from build123d import *

# Parameters (mm, degrees)
SKETCH3_R                = 48
SKETCH3_R_2              = 45
BOSS_EXTRUDE1_DEPTH      = 100
BOSS_EXTRUDE2_REACH      = 150.014
BOSS_EXTRUDE2_END_RADIUS = 48
SKETCH5_R                = 10
SKETCH6_R                = 10
BOSS_EXTRUDE3_DEPTH      = 40
SKETCH7_R                = 7
CUT_EXTRUDE1_DEPTH       = 55
SKETCH8_W                = 105
SKETCH8_H                = 105
SKETCH8_R                = 45
BOSS_EXTRUDE4_DEPTH      = 3
SKETCH9_W                = 105
SKETCH9_H                = 105
SKETCH9_W_2              = 100
SKETCH9_H_2              = 100
BOSS_EXTRUDE5_DEPTH      = 10


with BuildPart() as part:
    # Sketch3 → Boss-Extrude1 (new body)
    with BuildSketch(Plane(origin=(0, 0, 0), x_dir=(1, 0, 0), z_dir=(0, 1, 0))):
        with Locations(Location((0, 0, 0), (0, 0, 270))):
            Circle(SKETCH3_R)
        with Locations(Location((0, 0, 0), (0, 0, 270))):
            Circle(SKETCH3_R_2, mode=Mode.SUBTRACT)
    extrude(amount=BOSS_EXTRUDE1_DEPTH)

    # Boss-Extrude2: up to this cylinder (the profile starts outside it)
    boss_extrude2_end = Plane(origin=(0, 26.126098, 0), z_dir=(0, -1, 0)) * Cylinder(BOSS_EXTRUDE2_END_RADIUS, 397.028, mode=Mode.PRIVATE)
    # Sketch5 → Boss-Extrude2 (add, up to the surface)
    with BuildSketch(Plane(origin=(50, 0, 0), x_dir=(0, 0, -1), z_dir=(1, 0, 0)), mode=Mode.PRIVATE) as boss_extrude2_sk1:
        with Locations((0, 26.126097613)):
            Circle(SKETCH5_R)
    boss_extrude2_tool1 = extrude(boss_extrude2_sk1.sketch, amount=-BOSS_EXTRUDE2_REACH, mode=Mode.PRIVATE) - boss_extrude2_end
    add(boss_extrude2_tool1.solids().sort_by_distance((50, 26.126098, 0))[0])

    # Sketch6 → Boss-Extrude3 (add)
    with BuildSketch(Plane(origin=(50, 0, 0), x_dir=(0, 0, -1), z_dir=(1, 0, 0))):
        with Locations(Location((0, 25.974996965, 0), (0, 0, 179.567124411))):
            Circle(SKETCH6_R)
    extrude(amount=BOSS_EXTRUDE3_DEPTH)

    # Sketch7 → Cut-Extrude1 (cut)
    with BuildSketch(Plane(origin=(90, 0, 0), x_dir=(0, 0, -1), z_dir=(1, 0, 0))):
        with Locations((0, 26.126097613)):
            Circle(SKETCH7_R)
    extrude(amount=-CUT_EXTRUDE1_DEPTH, mode=Mode.SUBTRACT)

    # Sketch8 → Boss-Extrude4 (add)
    with BuildSketch(Plane(origin=(0, 100, 0), x_dir=(1, 0, 0), z_dir=(0, 1, 0))):
        Rectangle(SKETCH8_W, SKETCH8_H)
        with Locations(Location((0, 0, 0), (0, 0, 270))):
            Circle(SKETCH8_R, mode=Mode.SUBTRACT)
    extrude(amount=BOSS_EXTRUDE4_DEPTH)

    # Sketch9 → Boss-Extrude5 (add)
    with BuildSketch(Plane(origin=(0, 103, 0), x_dir=(1, 0, 0), z_dir=(0, 1, 0))):
        Rectangle(SKETCH9_W, SKETCH9_H)
        Rectangle(SKETCH9_W_2, SKETCH9_H_2, mode=Mode.SUBTRACT)
    extrude(amount=BOSS_EXTRUDE5_DEPTH)


solid = part.part
Work out the finished part from the listing and answer in its coordinate system (mm). A direction names the side the tool comes from. Round coordinates to 2 decimals unless told otherwise and drop trailing zeros. Write each loop counter-clockwise with the first axis right and the second up, starting at its lowest first coordinate (ties: lowest second). Pieces come first, ordered by that corner, then holes. Notation, with made-up numbers: (-27.75, 71) -> (-21.75, 71) arc R19 ccw to (-21.75, 105) -> close; hole circle Ø7 at (-35.75, 6). An arc over 180 degrees is marked (long way). Write each question's results on one line, items separated by ' | '.
Item 1: A cutting plane is placed at B-B, the plane z = 0. Determine the outline of the cut face in (x, y) (3 decimals).
Result set:
outline: (-52.5, 100) -> (-48, 100) -> (-48, 0) -> (-45, 0) -> (-45, 103) -> (-50, 103) -> (-50, 113) -> (-52.5, 113) -> close; (45, 0) -> (48, 0) -> (48, 16.126) -> (50, 16.126) -> (50, 15.975) -> (90, 15.975) -> (90, 19.126) -> (45, 19.126) -> close; (45, 33.126) -> (90, 33.126) -> (90, 35.975) -> (50, 35.975) -> (50, 36.126) -> (48, 36.126) -> (48, 100) -> (52.5, 100) -> (52.5, 113) -> (50, 113) -> (50, 103) -> (45, 103) -> close
Item 2: Which of the six approach directions +Z, -Z, +X, -X, +Y, -Y give full straight-line access (tool end or side, diameter ignored) to faces 4 (the face through (-1, 108, 50)), 5 (the face through (67.545, 19.293, 1.517)), 6 (the face through (-1, 106, -52.5))?
Result set:
face 4: +Y | face 5: +X | face 6: -Z, +X, -X, +Y, -Y
Item 3: A cutting plane is placed at A-A, the plane x = 0. Determine the outline of the cut face in (y, z).
Result set:
outline: (0, -48) -> (100, -48) -> (100, -52.5) -> (113, -52.5) -> (113, -50) -> (103, -50) -> (103, -45) -> (0, -45) -> close; (0, 45) -> (103, 45) -> (103, 50) -> (113, 50) -> (113, 52.5) -> (100, 52.5) -> (100, 48) -> (0, 48) -> close
Item 4: The mould has two halves that part along Y. Classify faces 1 (the face through (48.83, 22.3, -9.24)), 2 (the face through (50, 108, 1)), 3 (the face through (-14, 0, -43)): +Y half, -Y half, draft (parallel to the pull), parting line (faces both ways), or undercut.
Result set:
face 1: undercut | face 2: draft | face 3: -Y half
Item 5: Flat-ended cylindrical pins translate along their axes: P1, Ø1.5, axis at x = 63.5, z = 6, coming from the +Y side; P2, Ø5, axis at x = -33, y = 37.5, coming from the -Z side; P3, Ø3, axis at y = 81.5, z = -20, coming from the +X side. Find the tip coordinate at first contact, or state that the pin passes through.
Result set:
P1: y = 34.49 | P2: z = -37.06 | P3: x = 44.29
Item 6: A cutting plane is placed at C-C, the plane y = 105. Determine the outline of the cut face in (x, z).
Result set:
outline: (-52.5, -52.5) -> (52.5, -52.5) -> (52.5, 52.5) -> (-52.5, 52.5) -> close; hole (-50, -50) -> (50, -50) -> (50, 50) -> (-50, 50) -> close
Item 7: A cutting plane is placed at D-D, the plane z = -19.5. Determine the outline of the cut face in (x, y), plus the area to 3 significant figures.
Result set:
outline: (-52.5, 100) -> (-43.86, 100) -> (-43.86, 0) -> (-40.56, 0) -> (-40.56, 103) -> (-50, 103) -> (-50, 113) -> (-52.5, 113) -> close; (40.56, 0) -> (43.86, 0) -> (43.86, 100) -> (52.5, 100) -> (52.5, 113) -> (50, 113) -> (50, 103) -> (40.56, 103) -> close | area: 783 mm^2
Item 8: Find the intervals of material crossed by line 1 along Z through (x, y) = (11, 105); line 2 along Y through (x, z) = (78, 0.5); line 3 along X through (y, z) = (68, 0), in increasing order. Write a range as [from, to].
Result set:
line 1: [-52.5, -50], [50, 52.5] | line 2: [15.99, 19.14], [33.11, 35.96] | line 3: [-48, -45], [45, 48]
